from build123d import *

# Parameters (mm, degrees)
BOSS_EXTRUDE1_DEPTH = 45
SKETCH2_W           = 220
SKETCH2_H           = 200
BOSS_EXTRUDE2_DEPTH = 10


with BuildPart() as part:
    # Sketch1 → Boss-Extrude1 (new body)
    with BuildSketch(Plane(origin=(0, 0, 0), x_dir=(1, 0, 0), z_dir=(0, 1, 0))):
        Polygon((-110, -100), (-110, 100), (110, 100), (110, 80), (-90, 80), (-90, -80), (110, -80), (110, -100), align=None)
    extrude(amount=BOSS_EXTRUDE1_DEPTH)

    # Sketch2 → Boss-Extrude2 (add)
    with BuildSketch(Plane(origin=(0, 0, 0), x_dir=(-1, 0, 0), z_dir=(0, -1, 0))):
        Rectangle(SKETCH2_W, SKETCH2_H)
    extrude(amount=BOSS_EXTRUDE2_DEPTH)


solid = part.part
Work out the finished part from the listing and answer in its coordinate system (mm). A direction names the side the tool comes from. Coordinates: 2 decimals unless noted, no trailing zeros. Loops run counter-clockwise (first coordinate to the right, second up) from the corner with the lowest first, then second, coordinate; pieces in that order, holes last. Notation, with made-up numbers: (15, 80) -> (65, 80) arc R29 ccw to (65, 105) -> close; hole circle Ø8 at (66, 52). An arc over 180 degrees is marked (long way). Write each question's results on one line, items separated by ' | '. Start each with the question number.
1) Consider line 1 along Z through (x, y) = (-49, 42); line 2 along Y through (x, z) = (-64.5, -38); line 3 along X through (y, z) = (27, 70.5). Determine where each line is inside the solid, lowest interval first.
2) Find section B-B on y = 30.5. Determine the outline of the cut face in (x, z).
3) Find section C-C on x = 71.5. Determine the outline of the cut face in (y, z).
4) Find section A-A on z = 27.5. Determine the outline of the cut face in (x, y).
5) The mould has two halves that part along Z. Classify faces 1 (the flat face through (11, 22, -80)), 2 (the flat face through (2, 18, -100)), 3 (the flat face through (2, -10, -1)): pulls with the +Z half, pulls with the -Z half, needs draft (parallel to the pull), parting line crosses it, or undercut.
6) A flat-ended cylindrical pin translates along its axis: P1, Ø6, axis at x = -2, z = -59, coming from the +Y side. Find the tip coordinate at first contact, or state that the pin passes through.
7) For faces 4 (the flat face through (11, 0, -1)), 5 (the flat face through (-110, 18, 1)), determine the directions among +Z, -Z, +X, -X, +Y, -Y from which every point of the face is accessible in a straight line to the end or side of a thin tool.
Response values:
1) line 1: z = -100 to -80, 80 to 100 | line 2: y = -10 to 0 | line 3: x = -110 to -90
2) outline: (-110, -100) -> (110, -100) -> (110, -80) -> (-90, -80) -> (-90, 80) -> (110, 80) -> (110, 100) -> (-110, 100) -> close
3) outline: (-10, -100) -> (45, -100) -> (45, -80) -> (0, -80) -> (0, 80) -> (45, 80) -> (45, 100) -> (-10, 100) -> close
4) outline: (-110, -10) -> (110, -10) -> (110, 0) -> (-90, 0) -> (-90, 45) -> (-110, 45) -> close
5) face 1: undercut | face 2: pulls with the -Z half | face 3: needs draft
6) P1: stops at y = 0
7) face 4: +X, +Y | face 5: +Z, -Z, -X, +Y, -Y
